Build history of the part. All positions in model axes, mm. Face numbers are marked on the shaded views. A direction names the side the tool comes from. Give positions to 0.01 mm unless a question says otherwise; leave off trailing zeros. Order: outer loops, then holes, each group sorted by start corner. A loop starts at its lowest first (then second) coordinate and runs counter-clockwise, first axis right, second up. Notation, with made-up numbers: (81, 16) -> (116, 16) arc R22 cw to (116, 23) -> close; hole circle Ø6 at (36.5, 79). An arc over 180 degrees is marked (long way). Use a Markdown table: item, result. Add a question column.
```python
from build123d import *

# Parameters (mm, degrees)
F0_W     = 76.2
F0_H     = 76.2
F1_DEPTH = 25.4
F2_W     = 25.4
F2_H     = 25.4
F3_DEPTH = 25.4
F4_W     = 25.4
F4_H     = 25.4
F5_DEPTH = 12.7
F6_W     = 25.4
F6_H     = 25.4
F7_DEPTH = 50.8
F8_W     = 25.4
F8_H     = 25.4
F9_DEPTH = 38.1


with BuildPart() as f1:
    # F0 (on Top) → F1 (new body)
    with BuildSketch(Plane.XY):
        with Locations((-7.212972, 17.6349)):
            Rectangle(F0_W, F0_H)
    extrude(amount=F1_DEPTH)

    # F2 (on face) → F3 (join)
    with BuildSketch(Plane(origin=(0, 0, 0), x_dir=(1, 0, 0), z_dir=(0, 0, -1))):
        with Locations((-32.612972, -43.0349)):
            Rectangle(F2_W, F2_H)
    extrude(amount=F3_DEPTH)

    # F4 (on face) → F5 (join)
    with BuildSketch(Plane(origin=(0, 0, 0), x_dir=(1, 0, 0), z_dir=(0, 0, -1))):
        with Locations((-32.612972, 7.7651)):
            Rectangle(F4_W, F4_H)
    extrude(amount=F5_DEPTH)

    # F6 (on face) → F7 (join)
    with BuildSketch(Plane(origin=(0, 0, 0), x_dir=(1, 0, 0), z_dir=(0, 0, -1))):
        with Locations((18.187028, 7.7651)):
            Rectangle(F6_W, F6_H)
    extrude(amount=F7_DEPTH)

    # F8 (on face) → F9 (join)
    with BuildSketch(Plane(origin=(0, 0, 0), x_dir=(1, 0, 0), z_dir=(0, 0, -1))):
        with Locations((18.187028, -43.0349)):
            Rectangle(F8_W, F8_H)
    extrude(amount=F9_DEPTH)


solid = f1.part
```
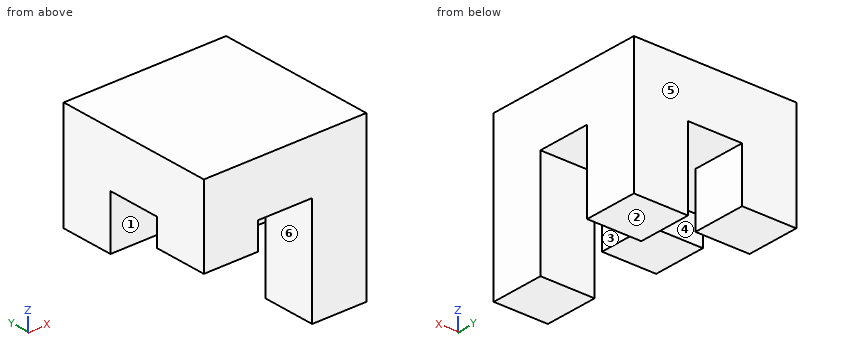
(1) Tool access for the marked faces 1, 2 and 3: list every direction of +Z, -Z, +X, -X, +Y, -Y with a clear straight run to the whole face (end or side of a thin tool).
(2) Pin check, flat tips, straight feed: pin 1 Ø20.5 at (y, z) = (-4, -25.5) entering from -X; pin 2 Ø1 at (x, z) = (4, -2) entering from -Y. Stop position of each tip, or through.
(3) Band-saw the part on D-D on y = 37. Give the cut face in (x, z), plus the area to 3 significant figures.
(4) Mould opens along Y. For the marked faces 4, 5 and 6 say: released by +Y, released by -Y, zero draft, split by the parting line, or undercut.
(5) Band-saw the part on C-C on z = -6.5. Give the cut face in (x, y).
(6) Band-saw the part on B-B on x = 20. Give the cut face in (y, z), plus the area to 3 significant figures.
(7) Wall check: probe 1 along X at (y, z) = (-13, -3.5); probe 2 along Y at (x, z) = (11, -32); probe 3 along Z at (x, y) = (20, 32). Give the ranges that are in metal, low to high.
(8) Band-saw the part on A-A on z = -32. Give the cut face in (x, y), plus the area to 3 significant figures.
Response:
| question | item | result |
|---|---|---|
| 1 | face 1 | -Z, +X, -X |
| 1 | face 2 | -Z, +X, -X, +Y |
| 1 | face 3 | -Z, +Y, -Y |
| 2 | pin 1 | stops at x = 5.49 |
| 2 | pin 2 | passes through |
| 3 | outline | (-45.31, -25.4) -> (-19.91, -25.4) -> (-19.91, 0) -> (5.49, 0) -> (5.49, -38.1) -> (30.89, -38.1) -> (30.89, 25.4) -> (-45.31, 25.4) -> close |
| 3 | area | 3,550 mm² |
| 4 | face 4 | undercut |
| 4 | face 5 | released by +Y |
| 4 | face 6 | zero draft |
| 5 | outline | (-45.31, -20.47) -> (-19.91, -20.47) -> (-19.91, 4.93) -> (-45.31, 4.93) -> close; (-45.31, 30.33) -> (-19.91, 30.33) -> (-19.91, 55.73) -> (-45.31, 55.73) -> close; (5.49, -20.47) -> (30.89, -20.47) -> (30.89, 4.93) -> (5.49, 4.93) -> close; (5.49, 30.33) -> (30.89, 30.33) -> (30.89, 55.73) -> (5.49, 55.73) -> close |
| 6 | outline | (-20.47, -50.8) -> (4.93, -50.8) -> (4.93, 0) -> (30.33, 0) -> (30.33, -38.1) -> (55.73, -38.1) -> (55.73, 25.4) -> (-20.47, 25.4) -> close |
| 6 | area | 4,190 mm² |
| 7 | probe 1 | x = -45.31 to -19.91, 5.49 to 30.89 |
| 7 | probe 2 | y = -20.47 to 4.93, 30.33 to 55.73 |
| 7 | probe 3 | z = -38.1 to 25.4 |
| 8 | outline | (5.49, -20.47) -> (30.89, -20.47) -> (30.89, 4.93) -> (5.49, 4.93) -> close; (5.49, 30.33) -> (30.89, 30.33) -> (30.89, 55.73) -> (5.49, 55.73) -> close |
| 8 | area | 1,290 mm² |
